Input: part model. Units: mm. Frame: model coordinates. A direction names the side the tool comes from. Give positions to 0.01 mm unless a question says otherwise; leave off trailing zeros. Write each loop counter-clockwise with the first axis right and the second up, starting at its lowest first coordinate (ties: lowest second). Pieces come first, ordered by that corner, then holes. Notation, with made-up numbers: (-3, -35.5) -> (3, -35.5) arc R22 ccw to (3, -13.5) -> close; hole circle Ø1 at (85, -7.5). An arc over 180 degrees is marked (long way). Return JSON: item names as keys, results as strings. Group by question number.
Item 1: Section D-D, the plane x = 8.75. Return loops of the section in (y, z) (3 decimals), then the cut area to 3 significant figures.
Item 2: Pin query (flat end, axial travel): P1, Ø1.5, axis at y = 49.5, z = 2.5, coming from the -X side (3 decimals); P2, Ø1.5, axis at y = 48, z = 2.5, coming from the +X side. Return the tip coordinate at first contact, or that it passes through.
Item 3: Mould query, pull axis Y, two halves, no side actions, for faces 1 (the face through (9.5, 41.5, 1.6)), 2 (the face through (0, 27.517, 2)), 3 (the face through (0, 54.949, 2)). Classes: released by +Y, released by -Y, zero draft, split by the parting line, or undercut.
Item 4: Section A-A, the plane z = 2.15. Return loops of the section in (x, y), then the cut area to 3 significant figures.
Item 5: Section C-C, the plane x = 1. Return loops of the section in (y, z) (3 decimals).
Item 6: Set-up query: faces 4 (the face through (-11.349, 38.434, 1.565)), 5 (the face through (10.862, 44.765, 1.565)), 6 (the face through (-10.817, 44.762, 1.565)), 7 (the face through (-12.26, 47.01, 1.57)). Return all of +Z, -Z, +X, -X, +Y, -Y with unobstructed straight access to the full face (end or side cutting, diameter ignored); none if empty.
Item 7: Section B-B, the plane y = 32.25. Return loops of the section in (x, z) (3 decimals).
Item 8: Line query: line 1 (Y direction, x = 0, z = 0.3); line 2 (Y direction, x = -6, z = 2.5); line 3 (X direction, y = 49.25, z = 2). Output: solid intervals per line, ascending. Write a range as [from, to].
from build123d import *

# Parameters (mm, degrees)
BOSS_EXTRUDE1_DEPTH = 3.175
CAVITY1_DEPTH       = 3.175


# Read off the part's stored shape, not the designer's step: Cavity1
with BuildPart() as part:
    # Sketch1 → Boss-Extrude1 (new body)
    with BuildSketch(Plane.XY):
        with BuildLine():
            Line((-6.901112522, 27.516666667), (0, 27.516666667))
            Line((0, 27.516666667), (0, 29.368749958))
            ThreePointArc((0, 29.368749958), (-2.38125, 31.749999958), (0, 34.131249958))
            Line((0, 34.131249958), (0, 48.418749958))
            ThreePointArc((0, 48.418749958), (-2.38125, 50.799999958), (0, 53.181249958))
            Line((0, 53.181249958), (0, 54.948666667))
            Line((0, 54.948666667), (-5.767881753, 54.948666667))
            ThreePointArc((-5.767881753, 54.948666667), (-10.082386674, 53.257802562), (-12.099177736, 49.085689435))
            Line((-12.099177736, 49.085689435), (-13.232408505, 34.353689435))
            ThreePointArc((-13.232408505, 34.353689435), (-11.560248417, 29.552161746), (-6.901112522, 27.516666667))
        make_face()
        with BuildLine():
            Line((0, 29.368749958), (0, 27.516666667))
            Line((0, 27.516666667), (6.901112522, 27.516666667))
            ThreePointArc((6.901112522, 27.516666667), (11.560248417, 29.552161746), (13.232408505, 34.353689435))
            Line((13.232408505, 34.353689435), (12.099177736, 49.085689435))
            ThreePointArc((12.099177736, 49.085689435), (10.082386674, 53.257802562), (5.767881753, 54.948666667))
            Line((5.767881753, 54.948666667), (0, 54.948666667))
            Line((0, 54.948666667), (0, 53.181249958))
            ThreePointArc((0, 53.181249958), (1.683798023, 52.48379798), (2.38125, 50.799999958))
            ThreePointArc((2.38125, 50.799999958), (1.683798023, 49.116201935), (0, 48.418749958))
            Line((0, 48.418749958), (0, 34.131249958))
            ThreePointArc((0, 34.131249958), (1.683798023, 33.43379798), (2.38125, 31.749999958))
            ThreePointArc((2.38125, 31.749999958), (1.683798023, 30.066201935), (0, 29.368749958))
        make_face()
    extrude(amount=BOSS_EXTRUDE1_DEPTH)

    # Cavity1 outline → Cavity1 (cut)
    with BuildSketch(Plane.XY):
        Polygon((9.256633745, 44.641826042), (9.743656513, 38.310530059), (12.909304504, 38.554041443), (12.422281737, 44.885337426), align=None)
        Polygon((-12.909304504, 38.554041443), (-9.743656513, 38.310530059), (-9.256633745, 44.641826042), (-12.422281736, 44.885337426), align=None)
    extrude(amount=CAVITY1_DEPTH, mode=Mode.SUBTRACT)


solid = part.part
Answer below:
{
 "1": {"outline": "(27.792, 0) -> (54.205, 0) -> (54.205, 3.175) -> (27.792, 3.175) -> close", "area": "83.9 mm2"},
 "2": {"P1": "stops at x = -12.125", "P2": "stops at x = 12.24"},
 "3": {"face 1": "undercut", "face 2": "released by -Y", "face 3": "released by +Y"},
 "4": {"outline": "(-13.23, 34.35) arc R6.35 ccw to (-6.9, 27.52) -> (6.9, 27.52) arc R6.35 ccw to (13.23, 34.35) -> (12.91, 38.55) -> (9.74, 38.31) -> (9.26, 44.64) -> (12.42, 44.89) -> (12.1, 49.09) arc R6.35 ccw to (5.77, 54.95) -> (-5.77, 54.95) arc R6.35 ccw to (-12.1, 49.09) -> (-12.42, 44.89) -> (-9.26, 44.64) -> (-9.74, 38.31) -> (-12.91, 38.55) -> close; hole circle Ø4.76 at (0, 31.75); hole circle Ø4.76 at (0, 50.8)", "area": "586 mm2"},
 "5": {"outline": "(27.517, 0) -> (29.589, 0) -> (29.589, 3.175) -> (27.517, 3.175) -> close; (33.911, 0) -> (48.639, 0) -> (48.639, 3.175) -> (33.911, 3.175) -> close; (52.961, 0) -> (54.949, 0) -> (54.949, 3.175) -> (52.961, 3.175) -> close"},
 "6": {"face 4": "+Z, -Z", "face 5": "+Z, -Z, +X", "face 6": "+Z, -Z, -X", "face 7": "+Z, -Z, -X, +Y"},
 "7": {"outline": "(-13.042, 0) -> (-2.328, 0) -> (-2.328, 3.175) -> (-13.042, 3.175) -> close; (2.328, 0) -> (13.042, 0) -> (13.042, 3.175) -> (2.328, 3.175) -> close"},
 "8": {"line 1": "y = [27.52, 29.37], [34.13, 48.42], [53.18, 54.95]", "line 2": "y = [27.52, 54.94]", "line 3": "x = [-12.08, -1.81], [1.81, 12.08]"}
}
